Can you work these out from the model? Positions are in its coordinate system, mm. A direction names the side the tool comes from. Give positions to 0.01 mm unless a question says otherwise; leave off trailing zeros. Loops run counter-clockwise (first coordinate to the right, second up) from the corner with the lowest first, then second, coordinate; pieces in that order, holes last. Notation, with made-up numbers: (-6, 71.5) -> (26, 71.5) arc R22 cw to (26, 95.5) -> close; hole circle Ø8 at (-36.75, 61). An arc over 180 degrees is marked (long way). Return JSON: item names as keys, results as strings. Group by question number.
Q1. Suppose I cut it at D-D, the plane x = 11. Please give me the cut outline in (y, z), and give its area (3 significant figures).
Q2. Suppose I cut it at B-B, the plane y = 11. Please give me the cut outline in (x, z).
Q3. Suppose I cut it at C-C, the plane x = 106.5. Please give me the cut outline in (y, z).
Q4. Which directions (+Z, -Z, +X, -X, +Y, -Y) give clear straight access to the entire face, cutting with the end or side of a thin tool? Please do faces 4 (the cylindrical face through (-1.978, 6.591, -2.579)), 5 (the cylindrical face through (109, 30, -29)).
Q5. Thinking about a two-plate mould opening in Z: for faces 1 (the cylindrical face through (38.597, 30.255, 24.655)), 2 (the cylindrical face through (-22.136, 30.255, -25.807)), 3 (the cylindrical face through (0.66, 2.465, -14.985)), which applies, pulls with the +Z half, pulls with the -Z half, needs draft (parallel to the pull), parting line crosses it, or undercut?
Q6. Will these pins go through, and if not, where does the flat tip stop? pin 1 (5.5 mm diameter, centred on y = 27, z = 31, fed in from +X); pin 2 (4.5 mm diameter, centred on x = 38.5, z = 29, fed in from -Y); pin 3 (12 mm diameter, centred on x = 87.5, z = -2.5, fed in from +Y); pin 4 (8 mm diameter, centred on x = 4.5, z = 29, fed in from +Y).
Q7. I need wall thicknesses on line 1 along X through (y, z) = (6.75, 0); line 2 along Z through (x, y) = (30.5, 22); line 3 along Z through (x, y) = (108, 14). Which ranges of each line are inside material? Lowest first, please. Write a range as [from, to].
Q8. Suppose I cut it at A-A, the plane z = 0. Please give me the cut outline in (x, y), and give its area (3 significant figures).
```python
from build123d import *

# Parameters (mm, degrees)
SKETCH1_R           = 15
BOSS_EXTRUDE1_DEPTH = 5
BOSS_EXTRUDE2_DEPTH = 8
BOSS_EXTRUDE3_DEPTH = 35
SKETCH4_R           = 2.1
SKETCH4_R_2         = 3.25
CUT_EXTRUDE1_DEPTH  = 35
SKETCH5_R           = 2.5
BOSS_EXTRUDE4_DEPTH = 35


with BuildPart() as part:
    # Sketch1 → Boss-Extrude1 (new body)
    with BuildSketch(Plane(origin=(0, 0, 0), x_dir=(1, 0, 0), z_dir=(0, 1, 0))):
        with Locations(Location((0, 0, 0), (0, 0, 270))):
            Circle(SKETCH1_R)
    extrude(amount=BOSS_EXTRUDE1_DEPTH)

    # Sketch2 → Boss-Extrude2 (add)
    with BuildSketch(Plane(origin=(0, 5, 0), x_dir=(1, 0, 0), z_dir=(0, 1, 0))):
        with BuildLine():
            Line((0, -37), (143.3, -37))
            ThreePointArc((143.3, -37), (180.3, 0), (143.3, 37))
            Line((143.3, 37), (0, 37))
            ThreePointArc((0, 37), (-37, 0), (0, -37))
        make_face()
    extrude(amount=BOSS_EXTRUDE2_DEPTH)

    # Sketch3 → Boss-Extrude3 (add)
    with BuildSketch(Plane(origin=(0, 13, 0), x_dir=(1, 0, 0), z_dir=(0, 1, 0))):
        with BuildLine():
            Line((143.3, 37), (0, 37))
            ThreePointArc((0, 37), (-37, 0), (0, -37))
            Line((0, -37), (143.3, -37))
            ThreePointArc((143.3, -37), (180.3, 0), (143.3, 37))
        make_face()
        with BuildLine():
            ThreePointArc((0, 34), (-34, 0), (0, -34))
            Line((0, -34), (143.3, -34))
            ThreePointArc((143.3, -34), (177.3, 0), (143.3, 34))
            Line((143.3, 34), (0, 34))
        make_face(mode=Mode.SUBTRACT)
    extrude(amount=BOSS_EXTRUDE3_DEPTH)

    # Sketch4 → Cut-Extrude1 (cut)
    with BuildSketch(Plane(origin=(0, 13, 0), x_dir=(1, 0, 0), z_dir=(0, 1, 0))):
        with Locations(Location((-11, 0, 0), (0, 0, 270))):
            Circle(SKETCH4_R)
        with Locations(Location((0, 0, 0), (0, 0, 270))):
            Circle(SKETCH4_R_2)
        with Locations(Location((0, 10.995299238, 0), (0, 0, 270))):
            Circle(SKETCH4_R)
        with Locations(Location((11, 0, 0), (0, 0, 270))):
            Circle(SKETCH4_R)
        with Locations(Location((0, -11, 0), (0, 0, 270))):
            Circle(SKETCH4_R)
    extrude(amount=-CUT_EXTRUDE1_DEPTH, mode=Mode.SUBTRACT)

    # Sketch5 → Boss-Extrude4 (add)
    # profile 1 of 9: a face of its own
    with BuildSketch(Plane(origin=(0, 13, 0), x_dir=(1, 0, 0), z_dir=(0, 1, 0))):
        with BuildLine():
            Line((-29, 4.5), (-33.700890196, 4.5))
            ThreePointArc((-33.700890196, 4.5), (-34, 0), (-33.700890196, -4.5))
            Line((-33.700890196, -4.5), (-29, -4.5))
            ThreePointArc((-29, -4.5), (-24.5, 0), (-29, 4.5))
        make_face()
        with Locations(Location((-29, 0, 0), (0, 0, 270))):
            Circle(SKETCH5_R, mode=Mode.SUBTRACT)
    # profile 2 of 9: a face of its own
    with BuildSketch(Plane(origin=(0, 13, 0), x_dir=(1, 0, 0), z_dir=(0, 1, 0))):
        with BuildLine():
            Line((9, 34), (0, 34))
            Line((0, 34), (0, 29))
            ThreePointArc((0, 29), (4.5, 24.5), (9, 29))
            Line((9, 29), (9, 34))
        make_face()
        with Locations(Location((4.5, 29, 0), (0, 0, 270))):
            Circle(SKETCH5_R, mode=Mode.SUBTRACT)
    # profile 3 of 9: a face of its own
    with BuildSketch(Plane(origin=(0, 13, 0), x_dir=(1, 0, 0), z_dir=(0, 1, 0))):
        with BuildLine():
            Line((43, 34), (34, 34))
            Line((34, 34), (34, 29))
            ThreePointArc((34, 29), (38.5, 24.5), (43, 29))
            Line((43, 29), (43, 34))
        make_face()
        with Locations(Location((38.5, 29, 0), (0, 0, 270))):
            Circle(SKETCH5_R, mode=Mode.SUBTRACT)
    # profile 4 of 9: a face of its own
    with BuildSketch(Plane(origin=(0, 13, 0), x_dir=(1, 0, 0), z_dir=(0, 1, 0))):
        with BuildLine():
            Line((77, 34), (68, 34))
            Line((68, 34), (68, 29))
            ThreePointArc((68, 29), (72.5, 24.5), (77, 29))
            Line((77, 29), (77, 34))
        make_face()
        with Locations(Location((72.5, 29, 0), (0, 0, 270))):
            Circle(SKETCH5_R, mode=Mode.SUBTRACT)
    # profile 5 of 9: a face of its own
    with BuildSketch(Plane(origin=(0, 13, 0), x_dir=(1, 0, 0), z_dir=(0, 1, 0))):
        with BuildLine():
            Line((68, -29), (68, -34))
            Line((68, -34), (77, -34))
            Line((77, -34), (77, -29))
            ThreePointArc((77, -29), (72.5, -24.5), (68, -29))
        make_face()
        with Locations(Location((72.5, -29, 0), (0, 0, 270))):
            Circle(SKETCH5_R, mode=Mode.SUBTRACT)
    # profile 6 of 9: a face of its own
    with BuildSketch(Plane(origin=(0, 13, 0), x_dir=(1, 0, 0), z_dir=(0, 1, 0))):
        with BuildLine():
            Line((34, -29), (34, -34))
            Line((34, -34), (43, -34))
            Line((43, -34), (43, -29))
            ThreePointArc((43, -29), (38.5, -24.653460046), (34, -29))
        make_face()
        with Locations(Location((38.5, -29, 0), (0, 0, 270))):
            Circle(SKETCH5_R, mode=Mode.SUBTRACT)
    # profile 7 of 9: a face of its own
    with BuildSketch(Plane(origin=(0, 13, 0), x_dir=(1, 0, 0), z_dir=(0, 1, 0))):
        with BuildLine():
            Line((0, -29), (0, -34))
            Line((0, -34), (9, -34))
            Line((9, -34), (9, -29))
            ThreePointArc((9, -29), (4.5, -24.5), (0, -29))
        make_face()
        with Locations(Location((4.5, -29, 0), (0, 0, 270))):
            Circle(SKETCH5_R, mode=Mode.SUBTRACT)
    # profile 8 of 9: a face of its own
    with BuildSketch(Plane(origin=(0, 13, 0), x_dir=(1, 0, 0), z_dir=(0, 1, 0))):
        with BuildLine():
            Line((111, 34), (102, 34))
            Line((102, 34), (102, 29))
            ThreePointArc((102, 29), (106.5, 24.5), (111, 29))
            Line((111, 29), (111, 34))
        make_face()
        with Locations(Location((106.5, 29, 0), (0, 0, 270))):
            Circle(SKETCH5_R, mode=Mode.SUBTRACT)
    # profile 9 of 9: a face of its own
    with BuildSketch(Plane(origin=(0, 13, 0), x_dir=(1, 0, 0), z_dir=(0, 1, 0))):
        with BuildLine():
            Line((102, -29), (102, -34))
            Line((102, -34), (111, -34))
            Line((111, -34), (111, -29))
            ThreePointArc((111, -29), (106.5, -24.5), (102, -29))
        make_face()
        with Locations(Location((106.5, -29, 0), (0, 0, 270))):
            Circle(SKETCH5_R, mode=Mode.SUBTRACT)
    extrude(amount=BOSS_EXTRUDE4_DEPTH)


solid = part.part
```
Ans:
{
 "1": {"outline": "(0, -10.2) -> (5, -10.2) -> (5, -37) -> (48, -37) -> (48, -34) -> (13, -34) -> (13, -2.1) -> (0, -2.1) -> close; (0, 2.1) -> (13, 2.1) -> (13, 34) -> (48, 34) -> (48, 37) -> (5, 37) -> (5, 10.2) -> (0, 10.2) -> close", "area": "849 mm^2"},
 "2": {"outline": "(0, -37) -> (143.3, -37) arc R37 ccw to (143.3, 37) -> (0, 37) arc R37 ccw to start; hole circle Ø4.2 at (-11, 0); hole circle Ø6.5 at (0, 0); hole circle Ø4.2 at (0, -11); hole circle Ø4.2 at (0, 11); hole circle Ø4.2 at (11, 0)"},
 "3": {"outline": "(5, -37) -> (48, -37) -> (48, -31.5) -> (13, -31.5) -> (13, -26.5) -> (48, -26.5) -> (48, -24.5) -> (13, -24.5) -> (13, 24.5) -> (48, 24.5) -> (48, 26.5) -> (13, 26.5) -> (13, 31.5) -> (48, 31.5) -> (48, 37) -> (5, 37) -> close"},
 "4": {"face 4": "+Y, -Y", "face 5": "+Y"},
 "5": {"face 1": "undercut", "face 2": "undercut", "face 3": "parting line crosses it"},
 "6": {"pin 1": "stops at x = 167.19", "pin 2": "stops at y = 5", "pin 3": "stops at y = 13", "pin 4": "stops at y = 48"},
 "7": {"line 1": "x = [-37, -13.1], [-8.9, -3.25], [3.25, 8.9], [13.1, 180.3]", "line 2": "z = [-37, -34], [34, 37]", "line 3": "z = [-37, -31], [-27, -24.76], [24.76, 27], [31, 37]"},
 "8": {"outline": "(-37, 5) -> (-15, 5) -> (-15, 0) -> (-13.1, 0) -> (-13.1, 13) -> (-24.5, 13) -> (-24.5, 48) -> (-26.5, 48) -> (-26.5, 13) -> (-31.5, 13) -> (-31.5, 48) -> (-37, 48) -> close; (-8.9, 0) -> (-3.25, 0) -> (-3.25, 13) -> (-8.9, 13) -> close; (3.25, 0) -> (8.9, 0) -> (8.9, 13) -> (3.25, 13) -> close; (13.1, 0) -> (15, 0) -> (15, 5) -> (180.3, 5) -> (180.3, 48) -> (177.3, 48) -> (177.3, 13) -> (13.1, 13) -> close", "area": "2,060 mm^2"}
}
